Model file for the job. Use its own axes, mm. A direction names the side the tool comes from. Round coordinates to 2 decimals unless told otherwise and drop trailing zeros. Loops run counter-clockwise (first coordinate to the right, second up) from the corner with the lowest first, then second, coordinate; pieces in that order, holes last.
from build123d import *

# Parameters (mm, degrees)
BOSS_EXTRUDE1_DEPTH = 4
SKETCH4_R           = 4
BOSS_EXTRUDE3_DEPTH = 6
CUT_EXTRUDE1_DEPTH  = 6


with BuildPart() as part:
    # Sketch1 → Boss-Extrude1 (new body)
    with BuildSketch(Plane(origin=(0, 0, 0), x_dir=(1, 0, 0), z_dir=(0, 1, 0))):
        with BuildLine():
            Line((-9.972243623, -5), (0, -5))
            ThreePointArc((0, -5), (3.535533906, -3.535533906), (5, 0))
            Line((5, 0), (2.5, 0))
            ThreePointArc((2.5, 0), (0, -2.5), (-2.5, 0))
            Line((-2.5, 0), (-21, 0))
            ThreePointArc((-21, 0), (-25, -4), (-29, 0))
            Line((-29, 0), (-47.5, 0))
            ThreePointArc((-47.5, 0), (-50, -2.5), (-52.5, 0))
            Line((-52.5, 0), (-55, 0))
            ThreePointArc((-55, 0), (-53.535533906, -3.535533906), (-50, -5))
            Line((-50, -5), (-40.027756377, -5))
            Line((-40.027756377, -5), (-9.972243623, -5))
        make_face()
        with BuildLine():
            Line((2.5, 0), (5, 0))
            ThreePointArc((5, 0), (3.535533906, 3.535533906), (0, 5))
            Line((0, 5), (-9.972243623, 5))
            Line((-9.972243623, 5), (-25, 5))
            Line((-25, 5), (-40.027756377, 5))
            Line((-40.027756377, 5), (-50, 5))
            ThreePointArc((-50, 5), (-53.535533906, 3.535533906), (-55, 0))
            Line((-55, 0), (-52.5, 0))
            ThreePointArc((-52.5, 0), (-50, 2.5), (-47.5, 0))
            Line((-47.5, 0), (-29, 0))
            ThreePointArc((-29, 0), (-25, 4), (-21, 0))
            Line((-21, 0), (-2.5, 0))
            ThreePointArc((-2.5, 0), (0, 2.5), (2.5, 0))
        make_face()
        with BuildLine():
            ThreePointArc((-15.519245585, -6.679497057), (-12.87008511, -5.429079735), (-9.972243623, -5))
            Line((-9.972243623, -5), (-40.027756377, -5))
            ThreePointArc((-40.027756377, -5), (-37.12991489, -5.429079735), (-34.480754415, -6.679497057))
            Line((-34.480754415, -6.679497057), (-33.519245585, -7.320502943))
            ThreePointArc((-33.519245585, -7.320502943), (-30.87008511, -8.570920265), (-27.972243623, -9))
            Line((-27.972243623, -9), (-22.027756377, -9))
            ThreePointArc((-22.027756377, -9), (-19.12991489, -8.570920265), (-16.480754415, -7.320502943))
            Line((-16.480754415, -7.320502943), (-15.519245585, -6.679497057))
        make_face()
        with BuildLine():
            Line((-25, 5), (-9.972243623, 5))
            ThreePointArc((-9.972243623, 5), (-12.87008511, 5.429079735), (-15.519245585, 6.679497057))
            Line((-15.519245585, 6.679497057), (-16.480754415, 7.320502943))
            ThreePointArc((-16.480754415, 7.320502943), (-19.12991489, 8.570920265), (-22.027756377, 9))
            Line((-22.027756377, 9), (-25, 9))
            Line((-25, 9), (-25, 5))
        make_face()
        with BuildLine():
            Line((-40.027756377, 5), (-25, 5))
            Line((-25, 5), (-25, 9))
            Line((-25, 9), (-27.972243623, 9))
            ThreePointArc((-27.972243623, 9), (-30.87008511, 8.570920265), (-33.519245585, 7.320502943))
            Line((-33.519245585, 7.320502943), (-34.480754415, 6.679497057))
            ThreePointArc((-34.480754415, 6.679497057), (-37.12991489, 5.429079735), (-40.027756377, 5))
        make_face()
    extrude(amount=BOSS_EXTRUDE1_DEPTH)

    # Sketch4 → Boss-Extrude3 (add)
    with BuildSketch(Plane(origin=(0, 4, 0), x_dir=(1, 0, 0), z_dir=(0, 1, 0))):
        with BuildLine():
            ThreePointArc((-15.521907779, 0), (-17.31867748, 5.552613483), (-22.027756377, 9))
            Line((-22.027756377, 9), (-27.972243623, 9))
            ThreePointArc((-27.972243623, 9), (-34.478092221, 0), (-27.972243623, -9))
            Line((-27.972243623, -9), (-22.027756377, -9))
            ThreePointArc((-22.027756377, -9), (-17.31867748, -5.552613483), (-15.521907779, 0))
        make_face()
        with Locations(Location((-25, 0, 0), (0, 0, 270))):
            Circle(SKETCH4_R, mode=Mode.SUBTRACT)
    extrude(amount=BOSS_EXTRUDE3_DEPTH)

    # Sketch5 → Cut-Extrude1 (cut)
    with BuildSketch(Plane(origin=(0, 0, -9), x_dir=(-1, 0, 0), z_dir=(0, 0, -1))):
        with BuildLine():
            ThreePointArc((26.65, 5), (26.166726189, 6.166726189), (25, 6.65))
            Line((25, 6.65), (25, 3.35))
            ThreePointArc((25, 3.35), (26.166726189, 3.833273811), (26.65, 5))
        make_face()
        with BuildLine():
            Line((25, 3.35), (25, 6.65))
            ThreePointArc((25, 6.65), (23.35, 5), (25, 3.35))
        make_face()
    extrude(amount=-CUT_EXTRUDE1_DEPTH, mode=Mode.SUBTRACT)


solid = part.part
Q1. Slice it at A-A on y = 1. Give the cut face in (x, z).
Q2. Slice it at D-D on x = -30.5. Give the cut face in (y, z).
Q3. Pull direction Z, two halves, no side cores. Call faces 5 (the face through (-37.169, 1.972, 5.417)), 6 (the face through (-12.831, 1.972, -5.417)), 7 (the face through (-52.31, 1.97, 0.96)): pulls with the +Z half, pulls with the -Z half, needs draft (parallel to the pull), parting line crosses it, or undercut.
Q4. Flat gauge pins, fed straight in: P1, Ø4.5, axis at x = -42.5, y = 3, coming from the +Z side; P2, Ø3, axis at x = -6.5, y = 2, coming from the -Z side; P3, Ø5.5, axis at x = -44, z = 0, coming from the +Y side. Where does each tip first touch, or does it go through?
Q5. Slice it at B-B on z = -1. Give the cut face in (x, y).
Q6. Slice it at C-C on x = 1.5. Give the cut face in (y, z).
Q7. Probe line 1 (X direction, y = 3.5, z = 0.25); line 2 (Z direction, x = 0, y = 1.9); line 3 (Z direction, x = -25, y = 8.25). List the from-to ranges inside material, lowest first.
Q8. Tool access for faces 1 (the face through (-45, 2, 5)), 2 (the face through (-25, 5, 9)), 3 (the face through (-45, 2, -5)), 4 (the face through (-5, 2, 5)): list every direction of +Z, -Z, +X, -X, +Y, -Y with a clear straight run to the whole face (end or side of a thin tool).
Reply:
1. outline: (-50, -5) - (-40.03, -5) arc R10 cw to (-34.48, -6.68) - (-33.52, -7.32) arc R10 ccw to (-27.97, -9) - (-22.03, -9) arc R10 ccw to (-16.48, -7.32) - (-15.52, -6.68) arc R10 cw to (-9.97, -5) - (0, -5) arc R5 ccw to (0, 5) - (-9.97, 5) arc R10 cw to (-15.52, 6.68) - (-16.48, 7.32) arc R10 ccw to (-22.03, 9) - (-27.97, 9) arc R10 ccw to (-33.52, 7.32) - (-34.48, 6.68) arc R10 cw to (-40.03, 5) - (-50, 5) arc R5 ccw to start; hole circle Ø5 at (-50, 0); hole circle Ø8 at (-25, 0); hole circle Ø5 at (0, 0)
2. outline: (0, -8.68) - (4, -8.68) - (4, -7.72) - (10, -7.72) - (10, 7.72) - (4, 7.72) - (4, 8.68) - (0, 8.68) - close
3. face 5: pulls with the +Z half
3. face 6: pulls with the -Z half
3. face 7: undercut
4. P1: stops at z = 5
4. P2: stops at z = -5
4. P3: stops at y = 4
5. outline: (-54.9, 0) - (-52.29, 0) - (-52.29, 4) - (-54.9, 4) - close; (-47.71, 0) - (-28.87, 0) - (-28.87, 10) - (-34.43, 10) - (-34.43, 4) - (-47.71, 4) - close; (-21.13, 0) - (-2.29, 0) - (-2.29, 4) - (-15.57, 4) - (-15.57, 10) - (-21.13, 10) - close; (2.29, 0) - (4.9, 0) - (4.9, 4) - (2.29, 4) - close
6. outline: (0, -4.77) - (4, -4.77) - (4, -2) - (0, -2) - close; (0, 2) - (4, 2) - (4, 4.77) - (0, 4.77) - close
7. line 1: x = -54.99 to -52.49, -47.51 to -28.99, -21.01 to -2.49, 2.49 to 4.99
7. line 2: z = -5 to -2.5, 2.5 to 5
7. line 3: z = -9 to -4, 4 to 9
8. face 1: +Z, -X, +Y, -Y
8. face 2: +Z, +X, -X, +Y, -Y
8. face 3: -Z, -X, +Y, -Y
8. face 4: +Z, +X, +Y, -Y
